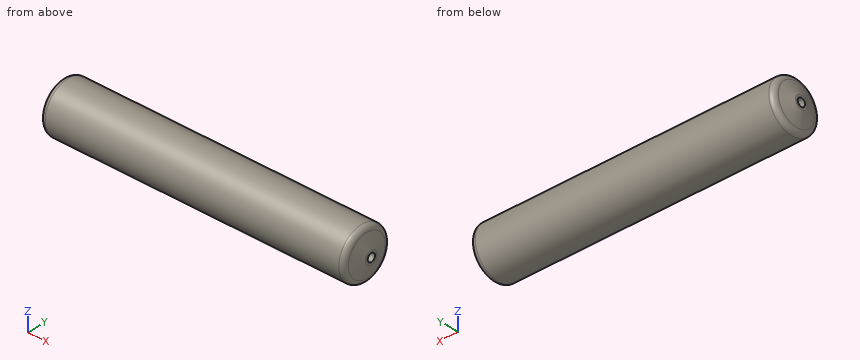
from build123d import *

# Parameters (mm, degrees)
ENL_V_MAT_EXTRU_1_DEPTH       = 0.1
BOSS_EXTRU_1_DEPTH            = 0.1
ENL_V_MAT_EXTRU_2_DEPTH       = 0.1
ENL_V_MAT_EXTRU_3_DEPTH       = 0.1
DIAM_TRE_DU_PER_AGE_8_0_8_1_D = 8


with BuildPart() as part:
    # Esquisse1 → Révolution1 (revolve)
    with BuildSketch(Plane.XY, mode=Mode.PRIVATE) as r_volution1_sk:
        with BuildLine():
            Line((-154.5, 6.4), (-154.5, 0))
            Line((-154.5, 0), (154.5, 0))
            Line((154.5, 0), (154.5, 6.4))
            Line((154.5, 6.4), (150, 20))
            ThreePointArc((150, 20), (148.535533906, 23.535533906), (145, 25))
            Line((145, 25), (-145, 25))
            ThreePointArc((-145, 25), (-148.535533906, 23.535533906), (-150, 20))
            Line((-150, 20), (-154.5, 6.4))
        make_face()
    revolve(r_volution1_sk.sketch.rotate(Axis((-154.5, 0, 0), (1, 0, 0)), 270), axis=Axis((-154.5, 0, 0), (1, 0, 0)))

    # Esquisse2 → Enlèv. mat.-Extru.1 (cut)
    with BuildSketch(Plane(origin=(154.5, 0, 0), x_dir=(0, 0, -1), z_dir=(1, 0, 0))):
        with BuildLine():
            Line((-0.220970869, 4.84375), (0.016600829, 4.84375))
            ThreePointArc((0.016600829, 4.84375), (0.407225829, 5.234375), (0.016600829, 5.625))
            Line((0.016600829, 5.625), (-0.533470869, 5.625))
            Line((-0.533470869, 5.625), (-0.533470869, 4.375))
            Line((-0.533470869, 4.375), (-0.220970869, 4.375))
            Line((-0.220970869, 4.375), (-0.220970869, 4.84375))
        make_face()
    extrude(amount=-ENL_V_MAT_EXTRU_1_DEPTH, mode=Mode.SUBTRACT)

    # Esquisse3 → Boss.-Extru.1 (add)
    with BuildSketch(Plane(origin=(154.4, 0, 0), x_dir=(0, 0, -1), z_dir=(1, 0, 0))):
        with BuildLine():
            Line((-0.220970869, 5.390625), (0.016600773, 5.390625))
            ThreePointArc((0.016600773, 5.390625), (0.172850773, 5.234375), (0.016600773, 5.078125))
            Line((0.016600773, 5.078125), (-0.220970869, 5.078125))
            Line((-0.220970869, 5.078125), (-0.220970869, 5.390625))
        make_face()
    extrude(amount=BOSS_EXTRU_1_DEPTH)

    # Esquisse4 → Enlèv. mat.-Extru.2 (cut)
    with BuildSketch(Plane(origin=(154.5, 0, 0), x_dir=(0, 0, -1), z_dir=(1, 0, 0))):
        Polygon((-1.001554062, 5.15625), (-1.314054062, 5.15625), (-1.314054062, 5.625), (-1.626554062, 5.625), (-1.626554062, 4.375), (-1.314054062, 4.375), (-1.314054062, 4.84375), (-1.001554062, 4.84375), (-1.001554062, 4.375), (-0.689054062, 4.375), (-0.689054062, 5.625), (-1.001554062, 5.625), align=None)
    extrude(amount=-ENL_V_MAT_EXTRU_2_DEPTH, mode=Mode.SUBTRACT)

    # Esquisse5 → Enlèv. mat.-Extru.3 (cut)
    with BuildSketch(Plane(origin=(154.5, 0, 0), x_dir=(0, 0, -1), z_dir=(1, 0, 0))):
        with BuildLine():
            ThreePointArc((1.626553937, 5.441941613), (0.5596125, 5), (1.626554062, 4.558058262))
            add(Edge.make_bspline(
                [(1.405583193, 4.779029131), (1.479240149, 4.705372175), (1.552897105, 4.631715218), (1.626554062, 4.558058262)],
                knots=[0, 0, 0, 0, 1, 1, 1, 1], degree=3))
            ThreePointArc((1.405583193, 4.779029131), (0.872112323, 5), (1.405583193, 5.220970869))
            add(Edge.make_bspline(
                [(1.626553937, 5.441941613), (1.552897022, 5.368284699), (1.479240107, 5.294627784), (1.405583193, 5.220970869)],
                knots=[0, 0, 0, 0, 1, 1, 1, 1], degree=3))
        make_face()
    extrude(amount=-ENL_V_MAT_EXTRU_3_DEPTH, mode=Mode.SUBTRACT)

    # Diamètre du perçage Ø8.0 (8)1 (through all)
    with Locations(Plane.ZY.offset(154.5)):
        with Locations((0, 0)):
            Hole(DIAM_TRE_DU_PER_AGE_8_0_8_1_D / 2)


solid = part.part
Model file for the job. Use its own axes, mm. Coordinates: 2 decimals unless noted, no trailing zeros. Loops run counter-clockwise (first coordinate to the right, second up) from the corner with the lowest first, then second, coordinate; pieces in that order, holes last. Notation, with made-up numbers: (66.25, -14) -> (82.25, -14) arc R14 ccw to (82.25, -1) -> close; hole circle Ø1 at (72, 41). An arc over 180 degrees is marked (long way). Use one line per item in the form item = value. Start each with the question number.
(1) Flat gauge pins, fed straight in: pin 1 (6 mm diameter, centred on x = 98.5, z = -5.5, fed in from +Y); pin 2 (1 mm diameter, centred on x = 120, y = 4.5, fed in from +Z); pin 3 (12 mm diameter, centred on x = -75.5, z = 17, fed in from -Y). Where does each tip first touch, or does it go through?
(2) Cut at A-A on y = 0. Give the cut face in (x, z).
(3) Probe probe 1 along Y at (x, z) = (140.5, 0.5) (3 decimals); probe 2 along X at (y, z) = (13, 14); probe 3 along Y at (x, z) = (-58, -21.5). List the from-to ranges inside material, lowest first. Write a range as from..to.
(4) Cut at B-B on x = 6.5. Give the cut face in (y, z).
Values:
q1.pin_1 = 24.87
q1.pin_2 = 24.68
q1.pin_3 = -22.45
q2.outline = (-154.5, -6.4) -> (-150, -20) arc R5 ccw to (-145, -25) -> (145, -25) arc R5 ccw to (150, -20) -> (154.5, -6.4) -> (154.5, -4) -> (-154.5, -4) -> close; (-154.5, 4) -> (154.5, 4) -> (154.5, 6.4) -> (150, 20) arc R5 ccw to (145, 25) -> (-145, 25) arc R5 ccw to (-150, 20) -> (-154.5, 6.4) -> close
q3.probe_1 = -24.995..-3.969, 3.969..24.995
q3.probe_2 = -150.3..150.3
q3.probe_3 = -12.76..12.76
q4.outline = circle Ø50 at (0, 0); hole circle Ø8 at (0, 0)
